```python
from build123d import *

# Parameters (mm, degrees)
F0_W        = 18.5
F0_H        = 13
F0_W_2      = 4.3
F0_W_3      = 3
F0_H_2      = 2.95
F1_DEPTH    = 10
F3_DEPTH    = 7
F4_T1_DEPTH = 35
F4_T3_DEPTH = 34.269322199
F0_H_3      = 5.9
F5_DEPTH    = 14
F6_R        = 5.5
F7_DEPTH    = 4
F8_SIZE     = 2


# Not quite as in the source:
# - a fillet or chamfer that OpenCascade refuses, or shapes differently, is made with other operations: its cross-section is extruded or revolved along the edge and cut away or added


with BuildPart() as f1:
    # F0 (on Top) → F1 (new body)
    with BuildSketch(Plane.XY):
        with Locations((5.190736489, 6.5)):
            Rectangle(F0_W, F0_H)
        with Locations((16.590736489, 6.5)):
            Rectangle(F0_W_2, F0_H)
        Polygon((14.440736489, 20.05), (14.440736489, 13), (18.740736489, 13), (18.740736489, 20.05), (15.740736489, 20.05), (15.740736489, 25.95), (18.740736489, 25.95), (18.740736489, 33), (14.440736489, 33), (14.440736489, 25.95), (14.440736489, 23), align=None)
        with BuildLine():
            Line((-4.059263511, 20.05), (-4.059263511, 13))
            Line((-4.059263511, 13), (14.440736489, 13))
            Line((14.440736489, 13), (14.440736489, 20.05))
            Line((14.440736489, 20.05), (11.440736489, 20.05))
            Line((11.440736489, 20.05), (11.440736489, 23))
            Line((11.440736489, 23), (9.590736489, 23))
            ThreePointArc((9.590736489, 23), (8.4904647177, 21.0659304563), (6.265736489, 21.0234183548))
            ThreePointArc((6.265736489, 21.0234183548), (4.0410082602, 21.0659304563), (2.940736489, 23))
            Line((2.940736489, 23), (-1.059263511, 23))
            Line((-1.059263511, 23), (-1.059263511, 20.05))
            Line((-1.059263511, 20.05), (-4.059263511, 20.05))
        make_face()
        with Locations((12.940736489, 21.525)):
            Rectangle(F0_W_3, F0_H_2)
        with Locations((12.940736489, 24.475)):
            Rectangle(F0_W_3, F0_H_2)
        with BuildLine():
            Line((-4.059263511, 33), (-4.059263511, 25.95))
            Line((-4.059263511, 25.95), (-1.059263511, 25.95))
            Line((-1.059263511, 25.95), (-1.059263511, 23))
            Line((-1.059263511, 23), (2.940736489, 23))
            ThreePointArc((2.940736489, 23), (4.0410082602, 24.9340695437), (6.265736489, 24.9765816452))
            ThreePointArc((6.265736489, 24.9765816452), (8.4904647177, 24.9340695437), (9.590736489, 23))
            Line((9.590736489, 23), (11.440736489, 23))
            Line((11.440736489, 23), (11.440736489, 25.95))
            Line((11.440736489, 25.95), (14.440736489, 25.95))
            Line((14.440736489, 25.95), (14.440736489, 33))
            Line((14.440736489, 33), (-4.059263511, 33))
        make_face()
        with BuildLine():
            Line((5.090736489, 23), (2.940736489, 23))
            ThreePointArc((2.940736489, 23), (4.0410082602, 21.0659304563), (6.265736489, 21.0234183548))
            ThreePointArc((6.265736489, 21.0234183548), (5.4066669452, 21.8502717712), (5.090736489, 23))
        make_face()
        with BuildLine():
            ThreePointArc((6.265736489, 24.9765816452), (4.0410082602, 24.9340695437), (2.940736489, 23))
            Line((2.940736489, 23), (5.090736489, 23))
            ThreePointArc((5.090736489, 23), (5.4066669452, 24.1497282288), (6.265736489, 24.9765816452))
        make_face()
    extrude(amount=F1_DEPTH)

    # F2 (on face) → F3 (cut)
    with BuildSketch(Plane.XZ):
        Polygon((2.940736489, 10), (0.940736489, 10), (0.940736489, 9), (1.940736489, 9), (1.940736489, 8), (0.940736489, 8), (0.940736489, 7), (1.940736489, 7), (1.940736489, 6), (0.940736489, 6), (0.940736489, 5), (1.940736489, 5), (1.940736489, 4), (0.940736489, 4), (0.940736489, 3), (1.940736489, 3), (1.940736489, 2), (0.940736489, 2), (0.940736489, 1), (1.940736489, 1), (1.940736489, 0), (2.940736489, 0), align=None)
        Polygon((14.940736489, 10), (12.940736489, 10), (12.940736489, 9), (13.940736489, 9), (13.940736489, 8), (12.940736489, 8), (12.940736489, 7), (13.940736489, 7), (13.940736489, 6), (12.940736489, 6), (12.940736489, 5), (13.940736489, 5), (13.940736489, 4), (12.940736489, 4), (12.940736489, 3), (13.940736489, 3), (13.940736489, 2), (12.940736489, 2), (12.940736489, 1), (13.940736489, 1), (13.940736489, 0), (14.940736489, 0), align=None)
    extrude(amount=-F3_DEPTH, mode=Mode.SUBTRACT)

    # F4: fillet of radius 5 on 4 edges, made by hand

    # F4_s2 → F4_t1 (cut)
    with BuildSketch(Plane.XY.offset(-12.5)):
        with BuildLine():
            ThreePointArc((-4.059263511, 28), (-2.594797417, 31.5355339059), (0.940736489, 33))
            Line((0.940736489, 33), (-4.059263511, 33))
            Line((-4.059263511, 33), (-4.059263511, 28))
        make_face()
        with BuildLine():
            ThreePointArc((0.940736489, 0), (-2.594797417, 1.4644660941), (-4.059263511, 5))
            Line((-4.059263511, 5), (-4.059263511, 0))
            Line((-4.059263511, 0), (0.940736489, 0))
        make_face()
        with BuildLine():
            ThreePointArc((13.740736489, 33), (17.2762703949, 31.5355339059), (18.740736489, 28))
            Line((18.740736489, 28), (18.740736489, 33))
            Line((18.740736489, 33), (13.740736489, 33))
        make_face()
    extrude(amount=F4_T1_DEPTH, mode=Mode.SUBTRACT)

    # F4_s4 → F4_t3 (cut)
    with BuildSketch(Plane.XY.offset(-12.1346610995)):
        with BuildLine():
            ThreePointArc((18.740736489, 4.8538644398), (17.677740426, 1.7716574383), (14.940736489, 0))
            Line((14.940736489, 0), (18.740736489, 0))
            Line((18.740736489, 0), (18.740736489, 4.8538644398))
        make_face()
    extrude(amount=F4_T3_DEPTH, mode=Mode.SUBTRACT)

    # F0 (on Top) → F5 (join)
    with BuildSketch(Plane.XY):
        with Locations((-2.559263511, 24.475)):
            Rectangle(F0_W_3, F0_H_2)
        with Locations((-2.559263511, 21.525)):
            Rectangle(F0_W_3, F0_H_2)
        with Locations((17.240736489, 23)):
            Rectangle(F0_W_3, F0_H_3)
    extrude(amount=F5_DEPTH)

    # F6 (on face) → F7 (cut)
    with BuildSketch(Plane(origin=(0, 0, 0), x_dir=(1, 0, 0), z_dir=(0, 0, -1))):
        with Locations((7.340736489, -23)):
            Circle(F6_R)
    extrude(amount=-F7_DEPTH, mode=Mode.SUBTRACT)

    # F8
    f8_edges = [f1.edges().sort_by_distance(p)[0] for p in [
        (1.840736, 23, 4),
    ]]
    chamfer(f8_edges, length=F8_SIZE)


solid = f1.part
```
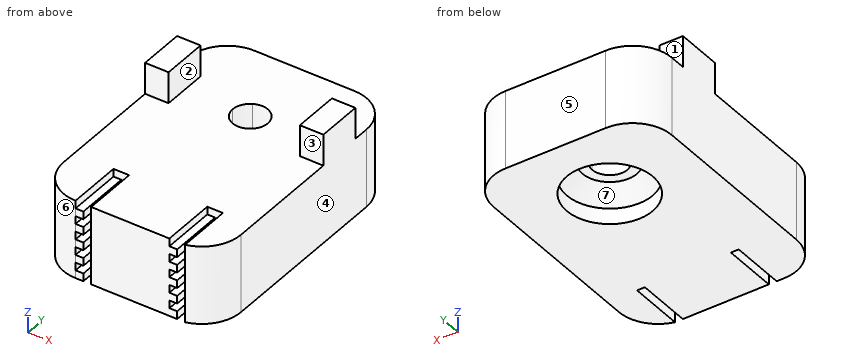
Here's how the part is built. I have some questions about the finished solid (model axes, mm). Face numbers are marked on the shaded views. A direction names the side the tool comes from. Coordinates: 2 decimals unless noted, no trailing zeros. Loops run counter-clockwise (first coordinate to the right, second up) from the corner with the lowest first, then second, coordinate; pieces in that order, holes last. Notation, with made-up numbers: M -38.5,-28.75 L -6.5,-28.75 A28 ccw -6.5,-9.75 Z; hole C -23.5,59.5 d8. An arc over 180 degrees is marked long. One line per item, written item: value.
1. Please list where these lines run through material, in increasing order: probe 1 along X at (y, z) = (23, 0.75); probe 2 along Z at (x, y) = (8.5, 17.5); probe 3 along Y at (x, z) = (9, 9.75).
Geometry says:
probe 1: x = -4.06 to 1.84, 12.84 to 18.74
probe 2: z = 0 to 10
probe 3: y = 0 to 21.48, 24.52 to 33
2. Imagine slicing it at B-B (x = -2.25). List the corners of the cut face in (y, z) for me.
Geometry says:
outline: M 1.15,0 L 31.85,0 L 31.85,10 L 25.95,10 L 25.95,14 L 20.05,14 L 20.05,10 L 1.15,10 Z
3. Thinking about a two-plate mould opening in Y: for the marked faces 4, 5, 6 and 7, which applies, +Y half, -Y half, draft (parallel to the pull), parting line (faces both ways), or undercut?
Geometry says:
face 4: draft
face 5: +Y half
face 6: -Y half
face 7: undercut
4. On a 3-axis mill with a long thin cutter (end or side, diameter ignored), from which of +Z, -Z, +X, -X, +Y, -Y can I reach the whole of each face in a straight line? I mean the marked faces 1, 2 and 3. Say none if no direction works.
Geometry says:
face 1: +Z, +X, -X, +Y
face 2: +Z, +Y, -Y
face 3: +Z, +X, -X, -Y
5. Imagine slicing it at C-C (y = 2). State how many separate pieces and enclosed holes the cut face has, and give its area (3 significant figures).
Geometry says:
separate pieces: 3
enclosed holes: 0
area: 179 mm2
6. Will these pins go through, and if not, where does the flat tip stop? pin 1 Ø4 at (x, y) = (11.5, 7) entering from -Z; pin 2 Ø1.5 at (x, y) = (4.5, 20.5) entering from -Z; pin 3 Ø4 at (x, y) = (10.5, 11.5) entering from +Z; pin 4 Ø1 at (y, z) = (11.5, 11.5) entering from +X.
Geometry says:
pin 1: stops at z = 0
pin 2: stops at z = 2.97
pin 3: stops at z = 10
pin 4: passes through
7. Imagine slicing it at A-A (z = 12.5). List the corners of the cut face in (x, y) for me, and give its area (3 significant figures).
Geometry says:
outline: M -4.06,20.05 L -1.06,20.05 L -1.06,25.95 L -4.06,25.95 Z; M 15.74,20.05 L 18.74,20.05 L 18.74,25.95 L 15.74,25.95 Z
area: 35.4 mm2
